Geometry: final body of the model. Coordinates: model frame, mm. Face numbers are marked on the shaded views. A direction names the side the tool comes from. Round coordinates to 2 decimals unless told otherwise and drop trailing zeros. Order: outer loops, then holes, each group sorted by start corner. A loop starts at its lowest first (then second) coordinate and runs counter-clockwise, first axis right, second up. Notation, with made-up numbers: (-37.5, -25) - (-0.5, -25) arc R20 ccw to (-0.5, 5) - close; hole circle Ø11 at (-22, -26.75). An arc over 180 degrees is marked (long way). Put each result on its own line as item: value. Start each with the question number.
(1) Section C-C (z = 2.75). Output: boundary loops of the cut face in (x, y), and give its area (3 significant figures).
(2) Section D-D (x = 1.5). Output: boundary loops of the cut face in (y, z).
(3) Material intervals for L1, parallel to X at y = 1, z = 2.55; L2, parallel to X at y = 0, z = 7.25; L3, parallel to Z at x = -5, y = -1, sorted ascending. Write a range as [from, to].
(4) Section A-A (x = -1.5). Output: boundary loops of the cut face in (y, z), and give its area (3 significant figures).
(5) Access query for the marked faces 1, 2, 3 and 4. Directions: +Z, -Z, +X, -X, +Y, -Y. A direction counts if a zero-diameter tool reaches every point of the face in a straight line with its end or side. Return the directions, or none.
(6) Section B-B (x = 4.75). Output: boundary loops of the cut face in (y, z).
(7) Pin query (flat end, axial travel): P1, Ø0.6, axis at x = 1, z = 8.5, coming from the +Y side (3 decimals); P2, Ø2.5, axis at y = -0.5, z = 8.5, coming from the -X side; P3, Ø1.1, axis at x = 10, z = -7, coming from the +Y side. Return the tip coordinate at first contact, or that it passes through.
(8) Pull-direction query (X, two-part tool) for the marked faces 5, 6 and 7; classes: released by +X, released by -X, zero draft, split by the parting line, or undercut.
from build123d import *

# Parameters (mm, degrees)
BOSS_EXTRU_1_DEPTH           = 3.1
CONG_1_R                     = 0.3
ENL_V_MAT_EXTRU_2_DEPTH      = 12.580803081
ENL_V_MAT_EXTRU_2_DEPTH_BACK = 12.580803081
ESQUISSE2_R                  = 1.1
BOSS_EXTRU_2_DEPTH           = 2
BOSS_EXTRU_3_DEPTH           = 0.3
CONG_2_R                     = 0.3
CONG_2_OF_SYM_TRIE1_R        = 0.3
BOSS_EXTRU_5_DEPTH           = 0.25
R_P_TITION_LIN_AIRE1_COUNT   = 2
R_P_TITION_LIN_AIRE1_PITCH   = 7.5
R_P_TITION_LIN_AIRE2_COUNT   = 2
R_P_TITION_LIN_AIRE2_PITCH   = 16.5


with BuildPart() as part:
    # Esquisse1 → Boss.-Extru.1 (new, symmetric)
    with BuildSketch(Plane(origin=(0, 0, 0), x_dir=(1, 0, 0), z_dir=(0, 1, 0))):
        Polygon((-9.95, -5.05), (-9.95, 5.05), (-0.95, 5.05), (-0.05, 4.4), (9.95, 4.4), (9.95, -5.05), align=None)
    extrude(amount=BOSS_EXTRU_1_DEPTH, both=True)

    # Congé1
    cong_1_edges = [part.edges().sort_by_distance(p)[0] for p in [
        (-9.95, 0, 5.05),
        (-9.95, 0, -5.05),
        (-0.95, 0, -5.05),
        (-0.05, 0, -4.4),
        (9.95, 0, -4.4),
        (9.95, 0, 5.05),
    ]]
    fillet(cong_1_edges, radius=CONG_1_R)

    # Esquisse2 → Enlèv. mat.-Extru.2 (cut, two sides: drawn at the far end of the back side and taken through both)
    with BuildSketch(Plane(origin=(0, 0, 0), x_dir=(1, 0, 0), z_dir=(0, 1, 0)).offset(-ENL_V_MAT_EXTRU_2_DEPTH_BACK)):
        with Locations(Location((-4.75, -2.55, 0), (0, 0, 90))):
            Circle(ESQUISSE2_R)
        with Locations(Location((4.75, -2.55, 0), (0, 0, 90))):
            Circle(ESQUISSE2_R)
    extrude(amount=ENL_V_MAT_EXTRU_2_DEPTH + ENL_V_MAT_EXTRU_2_DEPTH_BACK, mode=Mode.SUBTRACT)

    # Esquisse3 → Boss.-Extru.2 (add, symmetric)
    with BuildSketch(Plane(origin=(0, 0, 0), x_dir=(1, 0, 0), z_dir=(0, 1, 0))):
        with BuildLine():
            Line((-7.45, 5.05), (-7.45, 5.595028059))
            ThreePointArc((-7.45, 5.595028059), (-7.316741804, 5.916741804), (-6.995028059, 6.05))
            Line((-6.995028059, 6.05), (11.55, 6.05))
            Line((11.55, 6.05), (11.55, 5.75))
            Line((11.55, 5.75), (-6.9950313, 5.75))
            ThreePointArc((-6.9950313, 5.75), (-7.104610915, 5.704608624), (-7.15, 5.595028059))
            Line((-7.15, 5.595028059), (-7.15, 5.05))
            Line((-7.15, 5.05), (-7.45, 5.05))
        make_face()
    extrude(amount=BOSS_EXTRU_2_DEPTH, both=True)

    # Esquisse4 → Boss.-Extru.3 (add)
    with BuildSketch(Plane(origin=(0, 2, 0), x_dir=(1, 0, 0), z_dir=(0, 1, 0))):
        with BuildLine():
            Line((11.55, 5.75), (11.55, 8.97))
            ThreePointArc((11.55, 8.97), (9.725, 10.795), (7.9, 8.97))
            Line((7.9, 8.97), (7.9, 5.75))
            Line((7.9, 5.75), (11.55, 5.75))
        make_face()
    boss_extru_3 = extrude(amount=BOSS_EXTRU_3_DEPTH)

    # Congé2
    cong_2_edges = [part.edges().sort_by_distance(p)[0] for p in [
        (9.725, 2.3, -5.75),
    ]]
    fillet(cong_2_edges, radius=CONG_2_R)

    # Symétrie1: Boss.-Extru.3 across plane
    add(boss_extru_3.mirror(Plane.ZX))

    # Congé2 of Symétrie1
    cong_2_of_sym_trie1_edges = [part.edges().sort_by_distance(p)[0] for p in [
        (9.725, -2.3, -5.75),
    ]]
    fillet(cong_2_of_sym_trie1_edges, radius=CONG_2_OF_SYM_TRIE1_R)

    # Esquisse6 → Révolution1 (revolve)
    with BuildSketch(Plane.XY.offset(-8.97), mode=Mode.PRIVATE) as r_volution1_sk:
        with BuildLine():
            Line((9.725, 2), (9.725, -2))
            Line((9.725, -2), (11.69, -2))
            ThreePointArc((11.69, -2), (11.902132034, -1.912132034), (11.99, -1.7))
            Line((11.99, -1.7), (11.99, 1.7))
            ThreePointArc((11.99, 1.7), (11.902132034, 1.912132034), (11.69, 2))
            Line((11.69, 2), (9.725, 2))
        make_face()
    revolve(r_volution1_sk.sketch.rotate(Axis((9.725, 2, -8.97), (0, -1, 0)), 90), axis=Axis((9.725, 2, -8.97), (0, -1, 0)))

    # Esquisse7 → Boss.-Extru.5 (add, symmetric)
    with BuildSketch(Plane(origin=(8.45, 0, 0), x_dir=(0, 0, -1), z_dir=(1, 0, 0))):
        Polygon((-5.05, 1.6), (-5.05, -1.6), (-6.05, -1.6), (-6.05, -0.625), (-9.55, -0.625), (-9.55, 0.625), (-6.05, 0.625), (-6.05, 1.6), align=None)
    boss_extru_5 = extrude(amount=BOSS_EXTRU_5_DEPTH, both=True)

    # Répétition linéaire1: Boss.-Extru.5 ×2
    with Locations(*[(-i * R_P_TITION_LIN_AIRE1_PITCH, 0, 0) for i in range(1, R_P_TITION_LIN_AIRE1_COUNT)]):
        add(boss_extru_5)

    # Répétition linéaire2: Boss.-Extru.5 ×2
    with Locations(*[(-i * R_P_TITION_LIN_AIRE2_PITCH, 0, 0) for i in range(1, R_P_TITION_LIN_AIRE2_COUNT)]):
        add(boss_extru_5)


solid = part.part
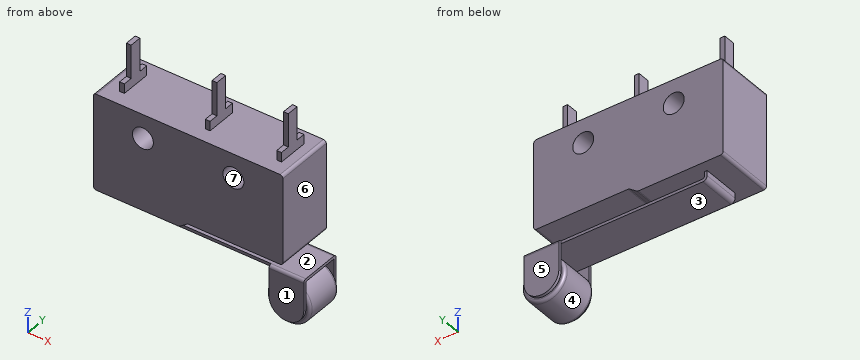
Checks:
1. outline: (-9.95, -3.1) - (-5.83, -3.1) - (-5.83, 3.1) - (-9.95, 3.1) - close; (-3.67, -3.1) - (3.67, -3.1) - (3.67, 3.1) - (-3.67, 3.1) - close; (5.83, -3.1) - (9.95, -3.1) - (9.95, 3.1) - (5.83, 3.1) - close
1. area: 96.6 mm²
2. outline: (-3.1, -4.4) - (3.1, -4.4) - (3.1, 5.05) - (-3.1, 5.05) - close; (-2, -6.05) - (2, -6.05) - (2, -5.75) - (-2, -5.75) - close
3. L1: x = [-9.95, -5.85], [-3.65, 3.65], [5.85, 9.95]
3. L2: x = [-8.3, -7.8], [0.7, 1.2], [8.2, 8.7]
3. L3: z = [-6.05, -5.75], [-5.05, 1.48], [3.62, 5.05]
4. outline: (-3.1, -5.05) - (3.1, -5.05) - (3.1, 5.05) - (-3.1, 5.05) - close; (-2, -6.05) - (2, -6.05) - (2, -5.75) - (-2, -5.75) - close
4. area: 63.8 mm²
5. face 1: -Z, +X, -X, -Y
5. face 2: +X, +Y, -Y
5. face 3: +X, -X
5. face 4: none
6. outline: (-3.1, -4.4) - (3.1, -4.4) - (3.1, 1.45) - (-3.1, 1.45) - close; (-3.1, 3.65) - (3.1, 3.65) - (3.1, 5.05) - (-3.1, 5.05) - close; (-2, -6.05) - (2, -6.05) - (2, -5.75) - (-2, -5.75) - close
7. P1: stops at y = 0.625
7. P2: stops at x = -8.3
7. P3: stops at y = 2.3
8. face 5: zero draft
8. face 6: released by +X
8. face 7: undercut
